For this review, take the finished solid that the model builds, in its own axes (mm). A direction names the side the tool comes from. Coordinates: 2 decimals unless noted, no trailing zeros. Write each loop counter-clockwise with the first axis right and the second up, starting at its lowest first coordinate (ties: lowest second). Pieces come first, ordered by that corner, then holes.
```python
from build123d import *

# Parameters (mm, degrees)
F0_W      = 90.986096
F0_H      = 41.3048
F1_DEPTH  = 25.4
F3_DEPTH  = 50.8
F4_W      = 7.798808
F4_H      = 5.902978
F5_DEPTH  = 101.6
F6_R      = 6.182282
F6_R_2    = 6.41324
F6_R_3    = 5.352968
F6_R_4    = 5.515412
F7_DEPTH  = 44.355903
F9_DEPTH  = 5.08
F10_W     = 45.493048
F10_H     = 6.787852
F11_DEPTH = 41.305801


with BuildPart() as f1:
    # F0 (on Top) → F1 (new body)
    with BuildSketch(Plane.XY):
        Rectangle(F0_W, F0_H)
    extrude(amount=F1_DEPTH)

    # F2 (on face) → F3 (cut)
    with BuildSketch(Plane.XZ.offset(20.6524)):
        Polygon((45.493048, 25.4), (0, 25.4), (45.493048, 0), align=None)
    extrude(amount=-F3_DEPTH, mode=Mode.SUBTRACT)

    # F4 (on face) → F5 (cut)
    with BuildSketch(Plane(origin=(-45.493048, 0, 0), x_dir=(0, -1, 0), z_dir=(-1, 0, 0))):
        with Locations((-1e-06, 22.448511)):
            Rectangle(F4_W, F4_H)
    extrude(amount=-F5_DEPTH, mode=Mode.SUBTRACT)

    # F6 (on face) → F7 (cut, through all)
    with BuildSketch(Plane(origin=(10.811308, 0, 19.363754), x_dir=(0.873128, 0, -0.487491), z_dir=(0.487491, 0, 0.873128))):
        with Locations((13.669491, -8.054403)):
            Circle(F6_R)
        with Locations((11.890859, 9.394533)):
            Circle(F6_R_2)
        with Locations((27.786525, 8.624507)):
            Circle(F6_R_3)
        with Locations((28.105455, -6.714204)):
            Circle(F6_R_4)
    extrude(amount=-F7_DEPTH, mode=Mode.SUBTRACT)

    # F8 (on face) → F9 (cut)
    with BuildSketch(Plane.XZ.offset(20.6524)):
        Polygon((14.875505, 17.094603), (14.875505, 0), (45.493048, 0), align=None)
    extrude(amount=-F9_DEPTH, mode=Mode.SUBTRACT)

    # F10 (on face) → F11 (cut, through all)
    with BuildSketch(Plane.XZ.offset(20.6524)):
        with Locations((-22.746524, 3.393926)):
            Rectangle(F10_W, F10_H)
    extrude(amount=-F11_DEPTH, mode=Mode.SUBTRACT)


solid = f1.part
```
1) Consider section B-B (y = -10). Give the boundary of the cut face in (x, z), then the cut area to 3 significant figures.
2) Consider section D-D (x = 37). Count the separate pieces of the cut face and the enclosed holes in it, then the cut area to 3 significant figures.
3) For L1, parallel to Y at x = -30, z = 22.5; L2, parallel to X at y = 5, z = 19.5; L3, parallel to Y at x = 11.5, z = 4, list the stretches that pass through material, from the lowest coordinate up.
4) Consider section A-A (z = 21.5). Give the boundary of the cut face in (x, y), then the cut area to 3 significant figures.
5) Tool access review of faces 1 (the face through (23, -15.572, 5)), 2 (the face through (-23, 0, 6.788)), 3 (the face through (-18, 3.899, 22)): name each direction out of +Z, -Z, +X, -X, +Y, -Y from which nothing blocks a thin tool from reaching the whole face with its end or side.
6) The part is to be moulded in two halves that separate along X. For faces 4 (the face through (28.736, -6.472, 5.117)), 5 (the face through (14.876, -18, 9)), 6 (the face through (-18, -3.899, 22)), 7 (the face through (-45.493, 0, 16)), say which applies: pulls with the +X half, pulls with the -X half, needs draft (parallel to the pull), parting line crosses it, or undercut.
7) Consider section C-C (x = -1.5). Give the boundary of the cut face in (y, z).
8) Clearance check with flat-ended pins moving along their axes: P1, Ø2.5, axis at y = -19, z = 6.5, coming from the +X side; P2, Ø8, axis at x = -18.5, y = 11, coming from the -Z side; P3, Ø4, axis at x = -30.5, y = -0.5, coming from the +Z side. State where each tip first meets the part, or that it passes through.
Results:
1. outline: (-45.49, 6.79) - (0, 6.79) - (0, 0) - (8.93, 0) - (17.62, 15.56) - (0, 25.4) - (-45.49, 25.4) - close; (22.38, 0) - (27.12, 0) - (31.48, 7.82) - (27.87, 9.84) - close; (37.26, 0) - (45.49, 0) - (39.22, 3.5) - close
1. area: 1,200 mm2
2. separate pieces: 3
2. enclosed holes: 0
2. area: 90.2 mm2
3. L1: y = -20.65 to -3.9, 3.9 to 20.65
3. L2: x = -45.49 to 10.57
3. L3: y = -20.65 to -10.72, -5.39 to 4.23, 14.56 to 20.65
4. outline: (-45.49, -20.65) - (6.99, -20.65) - (6.99, -3.9) - (-45.49, -3.9) - close; (-45.49, 3.9) - (6.99, 3.9) - (6.99, 20.65) - (-45.49, 20.65) - close
4. area: 1,760 mm2
5. face 1: +Z, -Z, +X, -Y
5. face 2: -Z, -X, +Y, -Y
5. face 3: +Z, +X, -X
6. face 4: undercut
6. face 5: pulls with the +X half
6. face 6: needs draft
6. face 7: pulls with the -X half
7. outline: (-20.65, 6.79) - (20.65, 6.79) - (20.65, 25.4) - (3.9, 25.4) - (3.9, 19.5) - (-3.9, 19.5) - (-3.9, 25.4) - (-20.65, 25.4) - close
8. P1: stops at x = 14.88
8. P2: stops at z = 6.79
8. P3: stops at z = 19.5
